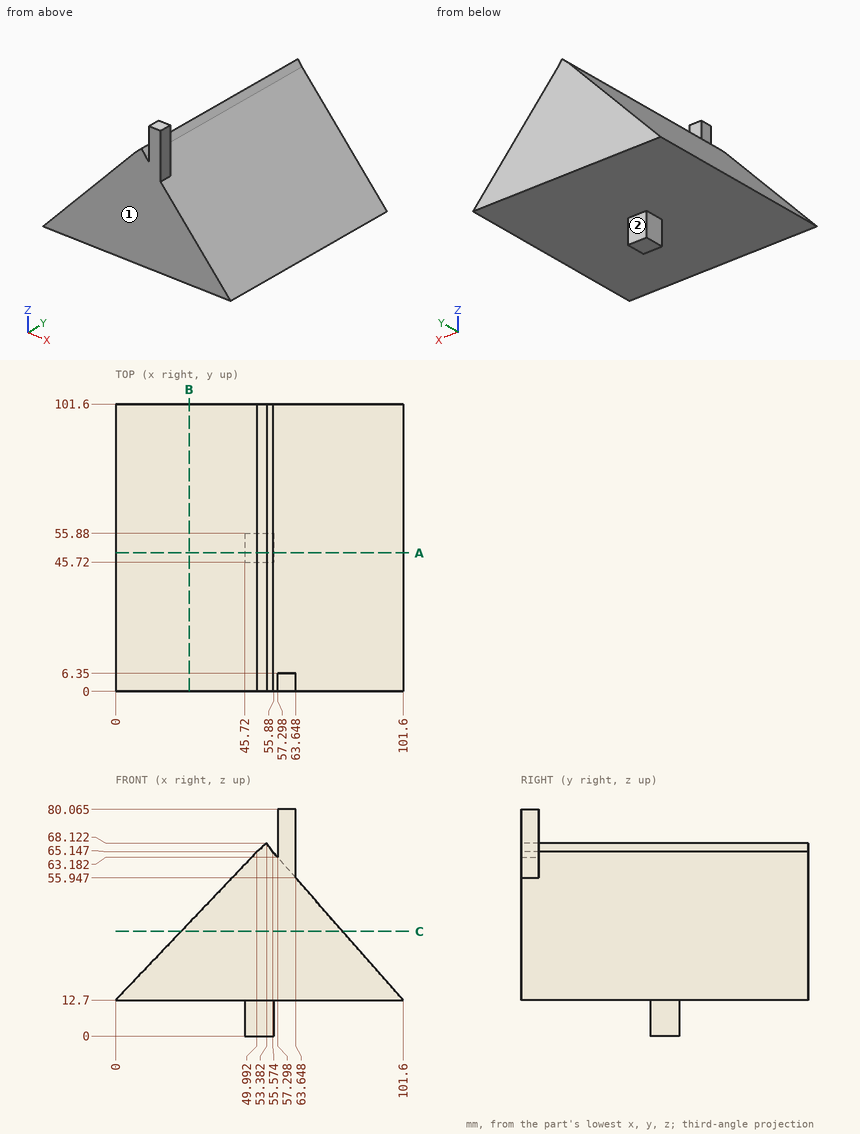
Geometry check sheet. Reference: drawing and pictorial views, mm from the part's lowest x, y, z. A direction names the side the tool comes from. Give positions to 0.01 mm unless a question says otherwise; leave off trailing zeros. Order: outer loops, then holes, each group sorted by start corner. A loop starts at its lowest first (then second) coordinate and runs counter-clockwise, first axis right, second up. Notation, with made-up numbers: (-36, 65) -> (16, 65) arc R29 ccw to (16, 89) -> close; hole circle Ø2 at (88, 29.5). An arc over 180 degrees is marked (long way). Write each question's results on one line, items separated by ' | '. Start each with the question number.
(1) Sectioned sample at C-C (z = 37). Enter the section's corners in (x, y) (1 decimal), plus the area to 3 significant figures.
(2) Sectioned sample at A-A (y = 49). Enter the section's corners in (x, z) (1 decimal), plus the area to 3 significant figures.
(3) Access from +Z, -Z, +X, -X, +Y, -Y to the whole of each face (thin tool, end or side, straight path). Record for the marked faces 1 and 2.
(4) Scan lines: line 1 (Y direction, x = 49, z = 7); line 2 (Y direction, x = 63, z = 60.5); line 3 (Z direction, x = 69, y = 61). Record each from-to range of solid material in increasing order.
(5) Sectioned sample at B-B (x = 26). Enter the section's corners in (y, z), plus the area to 3 significant figures.
(6) Gauge pin test, flat ends, axial feed: P1, Ø1.5, axis at x = 60, y = 48.5, coming from the -Z side; P2, Ø3, axis at x = 48.5, z = 5, coming from the +Y side; P3, Ø1, axis at y = 34, z = 27.5, coming from the -X side. Record the tip position at first contact, or that the pin passes through.
Answer below:
1) outline: (23.2, 0) -> (80.3, 0) -> (80.3, 101.6) -> (23.2, 101.6) -> close | area: 5,800 mm2
2) outline: (0, 12.7) -> (45.7, 12.7) -> (45.7, 0) -> (55.9, 0) -> (55.9, 12.7) -> (101.6, 12.7) -> (55.6, 65.1) -> (53.4, 68.1) -> (50, 65.1) -> close | area: 2,950 mm2
3) face 1: +Z, -Z, +X, -X, -Y | face 2: -Z, +X, -X, +Y
4) line 1: 45.72 to 55.88 | line 2: 0 to 6.35 | line 3: 12.7 to 49.85
5) outline: (0, 12.7) -> (101.6, 12.7) -> (101.6, 39.98) -> (0, 39.98) -> close | area: 2,770 mm2
6) P1: z = 12.7 | P2: y = 55.88 | P3: x = 13.63
